Design review of the part built by this model. Coordinates are the model's own, in mm. A direction names the side the tool comes from. Coordinates: 2 decimals unless noted, no trailing zeros. Order: outer loops, then holes, each group sorted by start corner. A loop starts at its lowest first (then second) coordinate and runs counter-clockwise, first axis right, second up. Notation, with made-up numbers: M -11,57 L 31,57 A19 ccw 31,81 Z; hole C 67.5,-27.75 d10. An arc over 180 degrees is marked long. Use CSV: the item, a comma, the result in double quotes.
```python
from build123d import *

# Parameters (mm, degrees)
SKETCH_1_R      = 15
EXTRUDE_1_DEPTH = 50
EXTRUDE_5_DEPTH = 10


with BuildPart() as part:
    # 草图1 → 凸台-拉伸1 (new body)
    with BuildSketch(Plane(origin=(0, 0, 0), x_dir=(1, 0, 0), z_dir=(0, 1, 0))):
        Circle(SKETCH_1_R)
    extrude(amount=EXTRUDE_1_DEPTH)

    # 草图6 → 凸台-拉伸5 (add, symmetric)
    with BuildSketch(Plane.XY):
        Polygon((-19.5, 0), (-6.5, -30), (-6.5, 0), align=None)
        Polygon((6.5, -30), (6.5, 0), (19.5, 0), align=None)
    extrude(amount=EXTRUDE_5_DEPTH, both=True)


solid = part.part
```
(1) The part is to be moulded in two halves that separate along X. For faces 1 (the face through (16, 0, 0)), 2 (the face through (-6.5, -15, 0)), 3 (the face through (13, -15, 0)), say which applies: pulls with the +X half, pulls with the -X half, needs draft (parallel to the pull), parting line crosses it, or undercut.
The answers:
face 1,"needs draft"
face 2,"undercut"
face 3,"pulls with the +X half"
(2) Add section B-B on z = 0. State the section outline as (x, y) points.
The answers:
outline,"M -19.5,0 L -6.5,-30 L -6.5,0 L 6.5,0 L 6.5,-30 L 19.5,0 L 15,0 L 15,50 L -15,50 L -15,0 Z"
(3) Add section C-C on x = 0. State the section outline as (y, z) points.
The answers:
outline,"M 0,-15 L 50,-15 L 50,15 L 0,15 Z"
(4) For faces 4 (the face through (6.5, -15, 0)), 5 (the face through (-10, -8, -10)), 6 (the face through (-14.985, 24.65, -0.66)), 7 (the face through (-10, -8, 10)), list the 3-axis set-ups (+Z, -Z, +X, -X, +Y, -Y) from which the entire face can be reached by the end or side of a thin tool; tool diameter is ignored.
The answers:
face 4,"+Z, -Z, -Y"
face 5,"-Z, +X, -X, -Y"
face 6,"+Y"
face 7,"+Z, +X, -X, -Y"
(5) Wall thickness on probe 1 along Y at (x, z) = (5, -7.75); probe 2 along Y at (x, z) = (16.5, -5.5); probe 3 along X at (y, z) = (-5.5, -1.5): over which ranges is each line inside the solid? List them lowest first.
The answers:
probe 1,"y = 0 to 50"
probe 2,"y = -6.92 to 0"
probe 3,"x = -17.12 to -6.5, 6.5 to 17.12"
(6) Add section A-A on y = -4.5. State the section outline as (x, z) points.
The answers:
outline,"M -17.55,-10 L -6.5,-10 L -6.5,10 L -17.55,10 Z; M 6.5,-10 L 17.55,-10 L 17.55,10 L 6.5,10 Z"
(7) Add section D-D on y = 22. State the section outline as (x, z) points, and give its area (3 significant figures).
The answers:
outline,"C 0,0 d30"
area,"707 mm2"
(8) Clearance check with flat-ended pins moving along their axes: P1, Ø10, axis at y = -21.5, z = -4, coming from the -X side; P2, Ø1, axis at x = 12, y = 29, coming from the -Z side; P3, Ø10.5, axis at x = 15, y = -10, coming from the -Z side. State where each tip first meets the part, or that it passes through.
The answers:
P1,"stops at x = -12.35"
P2,"stops at z = -9.63"
P3,"stops at z = -10"
